```python
from build123d import *

# Parameters (mm, degrees)
F0_W     = 101.6
F0_H     = 101.6
F1_DEPTH = 304.8
F2_R     = 4.7625
F3_DEPTH = 25.4
F4_R     = 4.7625
F5_DEPTH = 25.4


with BuildPart() as f1:
    # F0 (on Top) → F1 (new body)
    with BuildSketch(Plane.XY):
        Rectangle(F0_W, F0_H)
    extrude(amount=F1_DEPTH)

    # F2 (on face) → F3 (cut)
    with BuildSketch(Plane.XY.offset(304.8)):
        with Locations((-25.4, 25.4)):
            Circle(F2_R)
        with Locations((25.4, 25.4)):
            Circle(F2_R)
        with Locations((25.4, -25.4)):
            Circle(F2_R)
        with BuildLine():
            Line((0, 0), (0, -4.7625))
            ThreePointArc((0, -4.7625), (3.3675960454, -3.3675960454), (4.7625, 0))
            Line((4.7625, 0), (0, 0))
        make_face()
        with BuildLine():
            Line((0, 4.7625), (0, 0))
            Line((0, 0), (4.7625, 0))
            ThreePointArc((4.7625, 0), (3.3675960454, 3.3675960454), (0, 4.7625))
        make_face()
        with BuildLine():
            ThreePointArc((0, 4.7625), (-3.3675960454, 3.3675960454), (-4.7625, 0))
            Line((-4.7625, 0), (0, 0))
            Line((0, 0), (0, 4.7625))
        make_face()
        with BuildLine():
            ThreePointArc((-4.7625, 0), (-3.3675960454, -3.3675960454), (0, -4.7625))
            Line((0, -4.7625), (0, 0))
            Line((0, 0), (-4.7625, 0))
        make_face()
        with Locations((-25.4, -25.4)):
            Circle(F2_R)
    extrude(amount=-F3_DEPTH, mode=Mode.SUBTRACT)

    # F4 (on face) → F5 (cut)
    with BuildSketch(Plane(origin=(0, 0, 0), x_dir=(1, 0, 0), z_dir=(0, 0, -1))):
        with Locations((-25.4, 25.4)):
            Circle(F4_R)
        with Locations((25.4, 25.4)):
            Circle(F4_R)
        with Locations((25.4, -25.4)):
            Circle(F4_R)
        with Locations((-25.4, -25.4)):
            Circle(F4_R)
        with BuildLine():
            Line((0, 0), (-4.7625, 0))
            ThreePointArc((-4.7625, 0), (-3.3675960454, -3.3675960454), (0, -4.7625))
            Line((0, -4.7625), (0, 0))
        make_face()
        with BuildLine():
            Line((0, 0), (0, 4.7625))
            ThreePointArc((0, 4.7625), (-3.3675960454, 3.3675960454), (-4.7625, 0))
            Line((-4.7625, 0), (0, 0))
        make_face()
        with BuildLine():
            ThreePointArc((4.7625, 0), (3.3675960454, 3.3675960454), (0, 4.7625))
            Line((0, 4.7625), (0, 0))
            Line((0, 0), (4.7625, 0))
        make_face()
        with BuildLine():
            Line((4.7625, 0), (0, 0))
            Line((0, 0), (0, -4.7625))
            ThreePointArc((0, -4.7625), (3.3675960454, -3.3675960454), (4.7625, 0))
        make_face()
    extrude(amount=-F5_DEPTH, mode=Mode.SUBTRACT)


solid = f1.part
```
Build history of the part. All positions in model axes, mm. A direction names the side the tool comes from. Give positions to 0.01 mm unless a question says otherwise; leave off trailing zeros. Loops run counter-clockwise (first coordinate to the right, second up) from the corner with the lowest first, then second, coordinate; pieces in that order, holes last. Notation, with made-up numbers: (-16, 22) - (17, 22) arc R23 cw to (17, 57) - close; hole circle Ø4 at (73.25, 39). An arc over 180 degrees is marked (long way). Use a Markdown table: item, result.
(1) Pull direction Y, two halves, no side cores. Call faces 1 (the face through (-1, 50.8, 150)), 2 (the face through (11, 1, 304.8)), 3 (the face through (27.96, 21.384, 12.522)): +Y half, -Y half, draft (parallel to the pull), parting line (faces both ways), or undercut.
Taken from the geometry:
| item | result |
|---|---|
| face 1 | +Y half |
| face 2 | draft |
| face 3 | undercut |
(2) Wall check: line 1 along Y through (x, z) = (25, 20); line 2 along Y through (x, z) = (25.4, 290.75). Give the ranges that are in metal, low to high.
Taken from the geometry:
| item | result |
|---|---|
| line 1 | -50.8 to -30.15, -20.65 to 20.65, 30.15 to 50.8 |
| line 2 | -50.8 to -30.16, -20.64 to 20.64, 30.16 to 50.8 |
(3) Drop flat-ended pins along their axis: pin 1 Ø3 at (x, y) = (-2, 2) entering from +Z; pin 2 Ø8.5 at (x, y) = (25.4, -25.4) entering from -Z. Give the stop position or say it passes through.
Taken from the geometry:
| item | result |
|---|---|
| pin 1 | z = 279.4 |
| pin 2 | z = 25.4 |
(4) Which spindle directions (+Z, -Z, +X, -X, +Y, -Y) get a long thin tool onto all of the face, cutting with end or side? Do faces 4 (the face through (25, 25, 25.4)), 5 (the face through (11, 1, 0)), 6 (the face through (-25, 25, 279.4)). Say none if no direction does.
Taken from the geometry:
| item | result |
|---|---|
| face 4 | -Z |
| face 5 | -Z, +X, -X, +Y, -Y |
| face 6 | +Z |
(5) Band-saw the part on A-A (y = -25.4). Give the cut face in (x, z), and give its area (3 significant figures).
Taken from the geometry:
| item | result |
|---|---|
| outline | (-50.8, 0) - (-30.16, 0) - (-30.16, 25.4) - (-20.64, 25.4) - (-20.64, 0) - (20.64, 0) - (20.64, 25.4) - (30.16, 25.4) - (30.16, 0) - (50.8, 0) - (50.8, 304.8) - (30.16, 304.8) - (30.16, 279.4) - (20.64, 279.4) - (20.64, 304.8) - (-20.64, 304.8) - (-20.64, 279.4) - (-30.16, 279.4) - (-30.16, 304.8) - (-50.8, 304.8) - close |
| area | 30,000 mm2 |
